from build123d import *

# Parameters (mm, degrees)
SKETCH1_W           = 19.05
SKETCH1_H           = 31.75
SKETCH1_R           = 2.032
BOSS_EXTRUDE1_DEPTH = 25.4
SKETCH2_R           = 2.032
CUT_EXTRUDE1_DEPTH  = 45.901280605
FILLET1_R           = 1.190625


with BuildPart() as part:
    # Sketch1 → Boss-Extrude1 (new body)
    with BuildSketch(Plane.XY):
        with Locations((9.525, 15.875)):
            Rectangle(SKETCH1_W, SKETCH1_H)
        with Locations((4.7625, 26.9875)):
            Circle(SKETCH1_R, mode=Mode.SUBTRACT)
        with Locations((14.2875, 26.9875)):
            Circle(SKETCH1_R, mode=Mode.SUBTRACT)
        with Locations((4.7625, 4.7625)):
            Circle(SKETCH1_R, mode=Mode.SUBTRACT)
        with Locations((14.2875, 4.7625)):
            Circle(SKETCH1_R, mode=Mode.SUBTRACT)
    extrude(amount=BOSS_EXTRUDE1_DEPTH)

    # Sketch2 → Cut-Extrude1 (cut, through all)
    with BuildSketch(Plane.ZY):
        with Locations((17.960512242, 17.960512242)):
            Circle(SKETCH2_R)
    extrude(amount=-CUT_EXTRUDE1_DEPTH, mode=Mode.SUBTRACT)

    # Fillet1
    fillet1_edges = [part.edges().sort_by_distance(p)[0] for p in [
        (9.525, 31.75, 0),
        (19.05, 15.875, 0),
        (9.525, 0, 0),
        (0, 15.875, 0),
        (0, 31.75, 12.7),
        (19.05, 31.75, 12.7),
        (19.05, 0, 12.7),
        (0, 0, 12.7),
    ]]
    fillet(fillet1_edges, radius=FILLET1_R)


solid = part.part
Could you check a few things on this model? Use its own coordinates, in mm. Round coordinates to 2 decimals unless told otherwise and drop trailing zeros. Order: outer loops, then holes, each group sorted by start corner. A loop starts at its lowest first (then second) coordinate and runs counter-clockwise, first axis right, second up.
(1) Imagine slicing it at A-A (x = 13). Write out the boundary of the cut face in (y, z).
Response values:
outline: (0, 1.19) arc R1.19 ccw to (1.19, 0) - (3.19, 0) - (3.19, 25.4) - (0, 25.4) - close; (6.33, 0) - (25.42, 0) - (25.42, 25.4) - (6.33, 25.4) - close; (28.56, 0) - (30.56, 0) arc R1.19 ccw to (31.75, 1.19) - (31.75, 25.4) - (28.56, 25.4) - close; hole circle Ø4.06 at (17.96, 17.96)
(2) Please list where these lines run through material, in increasing order: line 1 along Y through (x, z) = (14.25, 1.25); line 2 along X through (y, z) = (4, 19); line 3 along Y through (x, z) = (15.5, 7.75).
Response values:
line 1: y = 0 to 2.73, 6.79 to 24.96, 29.02 to 31.75
line 2: x = 0 to 2.88, 6.65 to 12.4, 16.17 to 19.05
line 3: y = 0 to 3.13, 6.39 to 25.36, 28.62 to 31.75
(3) If we mould it in two halves opening along X, with no side actions, what happens to faces 1 (the cylindrical face through (4.32, 2.78, 12.52)), 2 (the flat face through (9, 16, 0)), 3 (the cylindrical face through (18.69, 0.34, 13.46)), 4 (the flat face through (0, 16, 13))? For each: released by +X, released by -X, zero draft, split by the parting line, or undercut.
Response values:
face 1: undercut
face 2: zero draft
face 3: released by +X
face 4: released by -X
(4) Imagine slicing it at C-C (z = 13.5). Write out the boundary of the cut face in (x, y), plus the area to 3 significant figures.
Response values:
outline: (0, 1.19) arc R1.19 ccw to (1.19, 0) - (17.86, 0) arc R1.19 ccw to (19.05, 1.19) - (19.05, 30.56) arc R1.19 ccw to (17.86, 31.75) - (1.19, 31.75) arc R1.19 ccw to (0, 30.56) - close; hole circle Ø4.06 at (4.76, 4.76); hole circle Ø4.06 at (4.76, 26.99); hole circle Ø4.06 at (14.29, 4.76); hole circle Ø4.06 at (14.29, 26.99)
area: 552 mm2
(5) Imagine slicing it at D-D (x = 15). Write out the boundary of the cut face in (y, z).
Response values:
outline: (0, 1.19) arc R1.19 ccw to (1.19, 0) - (2.86, 0) - (2.86, 25.4) - (0, 25.4) - close; (6.67, 0) - (25.08, 0) - (25.08, 25.4) - (6.67, 25.4) - close; (28.89, 0) - (30.56, 0) arc R1.19 ccw to (31.75, 1.19) - (31.75, 25.4) - (28.89, 25.4) - close; hole circle Ø4.06 at (17.96, 17.96)
(6) Imagine slicing it at B-B (y = 19.5). Write out the boundary of the cut face in (x, z), plus the area to 3 significant figures.
Response values:
outline: (0, 1.19) arc R1.19 ccw to (1.19, 0) - (17.86, 0) arc R1.19 ccw to (19.05, 1.19) - (19.05, 16.63) - (0, 16.63) - close; (0, 19.29) - (19.05, 19.29) - (19.05, 25.4) - (0, 25.4) - close
area: 433 mm2
